```python
from build123d import *

# Parameters (mm, degrees)
F0_R     = 9.525
F1_DEPTH = 7


with BuildPart() as f1:
    # F0 (on Top) → F1 (new body)
    with BuildSketch(Plane.XY):
        with BuildLine():
            ThreePointArc((-7.356254, 8.178357), (3.329824, 10.483905), (10.727142, 2.434838))
            Line((10.727142, 2.434838), (14.408928, 3.270526))
            ThreePointArc((14.408928, 3.270526), (15.252655, 10.351743), (20.379099, 15.309069))
            Line((20.379099, 15.309069), (14.740562, 40.150721))
            ThreePointArc((14.740562, 40.150721), (13.015163, 42.014748), (10.538168, 41.452522))
            Line((10.538168, 41.452522), (-8.102103, 24.198528))
            ThreePointArc((-8.102103, 24.198528), (-7.387937, 17.616196), (-10.676531, 11.869695))
            Line((-10.676531, 11.869695), (-7.356254, 8.178357))
        make_face()
        with Locations((6.842669, 22.233071)):
            Circle(F0_R, mode=Mode.SUBTRACT)
        with BuildLine():
            Line((-4.402173, -13.902461), (-3.320622, -10.486824))
            ThreePointArc((-3.320622, -10.486824), (-10.751566, -2.324615), (-7.356254, 8.178357))
            Line((-7.356254, 8.178357), (-10.676531, 11.869695))
            ThreePointArc((-10.676531, 11.869695), (-16.61004, 9.162756), (-23.01432, 10.395333))
            Line((-23.01432, 10.395333), (-41.654591, -6.85866))
            ThreePointArc((-41.654591, -6.85866), (-42.406186, -9.284914), (-40.680787, -11.148941))
            Line((-40.680787, -11.148941), (-16.55213, -18.617483))
            ThreePointArc((-16.55213, -18.617483), (-11.304982, -14.126767), (-4.402173, -13.902461))
        make_face()
        with Locations((-22.614271, -5.452181)):
            Circle(F0_R, mode=Mode.SUBTRACT)
        with BuildLine():
            ThreePointArc((10.727142, 2.434838), (10.931573, 1.225039), (11, 0))
            ThreePointArc((11, 0), (6.498968, -8.874876), (-3.320622, -10.486824))
            Line((-3.320622, -10.486824), (-4.402173, -13.902461))
            ThreePointArc((-4.402173, -13.902461), (1.09613, -17.999523), (2.859245, -24.625885))
            Line((2.859245, -24.625885), (26.987902, -32.094427))
            ThreePointArc((26.987902, -32.094427), (29.624289, -31.725007), (30.482894, -29.205125))
            Line((30.482894, -29.205125), (24.991316, -5.010931))
            ThreePointArc((24.991316, -5.010931), (18.227056, -2.752546), (14.408928, 3.270526))
            Line((14.408928, 3.270526), (10.727142, 2.434838))
        make_face()
        with Locations((15.648209, -17.212353)):
            Circle(F0_R, mode=Mode.SUBTRACT)
    extrude(amount=F1_DEPTH)


solid = f1.part
```
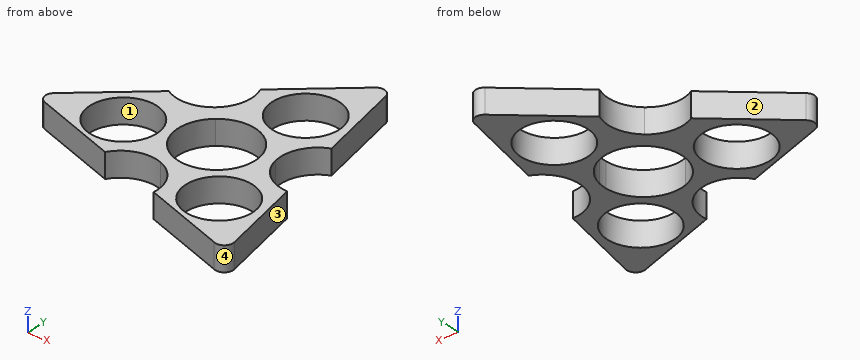
Build history of the part. All positions in model axes, mm. Face numbers are marked on the shaded views. Round coordinates to 2 decimals unless told otherwise and drop trailing zeros. Write each loop counter-clockwise with the first axis right and the second up, starting at its lowest first coordinate (ties: lowest second). Pieces come first, ordered by that corner, then holes. Notation, with made-up numbers: (76, 5) - (111, 5) arc R12 ccw to (111, 14) - close; hole circle Ø11 at (-10.75, 60). An arc over 180 degrees is marked (long way). Write each question's results on one line, items separated by ' | '. Start each with the question number.
Item 1: Mould opens along X. For the marked faces 1, 2, 3 and 4 say: pulls with the +X half, pulls with the -X half, needs draft (parallel to the pull), parting line crosses it, or undercut.
Item 2: Saw through at A-A (y = 18). Write the cut outline in (x, z), and give its area (3 significant figures).
Item 3: Saw through at C-C (z = 2.75). State how many separate pieces and enclosed holes the cut face has, and give its area (3 significant figures).
Item 4: Drop flat-ended pins along their axis: P1, Ø2, axis at x = -7, z = 4.5, coming from the -Y side; P2, Ø4, axis at y = -6.5, z = 2.5, coming from the +X side; P3, Ø1.5, axis at x = -24, z = 2, coming from the +Y side. Give the stop position or say it passes through.
Item 5: Saw through at B-B (x = -6). Write the cut outline in (y, z), and give its area (3 significant figures).
Item 6: Wall check: L1, parallel to X at y = -3, z = 5.25; L2, parallel to Y at x = 5.5, z = 6; L3, parallel to Y at x = 1.5, z = 2. Give the ranges that are in metal, low to high. Write a range as [from, to].
Item 7: Saw through at D-D (x = 18.5). Write the cut outline in (y, z), and give its area (3 significant figures).
Results are:
1) face 1: undercut | face 2: pulls with the -X half | face 3: pulls with the +X half | face 4: parting line crosses it
2) outline: (-7.32, 0) - (-1.69, 0) - (-1.69, 7) - (-7.32, 7) - close; (15.38, 0) - (19.77, 0) - (19.77, 7) - (15.38, 7) - close | area: 70.1 mm²
3) separate pieces: 1 | enclosed holes: 4 | area: 1,150 mm²
4) P1: stops at y = -13.53 | P2: stops at x = 25.78 | P3: stops at y = 10.18
5) outline: (-13.53, 0) - (-9.22, 0) - (-9.22, 7) - (-13.53, 7) - close; (9.22, 0) - (26.14, 0) - (26.14, 7) - (9.22, 7) - close | area: 149 mm²
6) L1: x = [-37.49, -31.82], [-13.41, -10.58], [10.58, 18.56] | L2: y = [-25.44, -9.53], [9.53, 12.8], [31.66, 36.79] | L3: y = [-18.65, -10.9], [10.9, 14.35], [30.12, 33.09]
7) outline: (-29.47, 0) - (-26.3, 0) - (-26.3, 7) - (-29.47, 7) - close; (-8.12, 0) - (-2.96, 0) - (-2.96, 7) - (-8.12, 7) - close; (14.21, 0) - (23.59, 0) - (23.59, 7) - (14.21, 7) - close | area: 124 mm²
